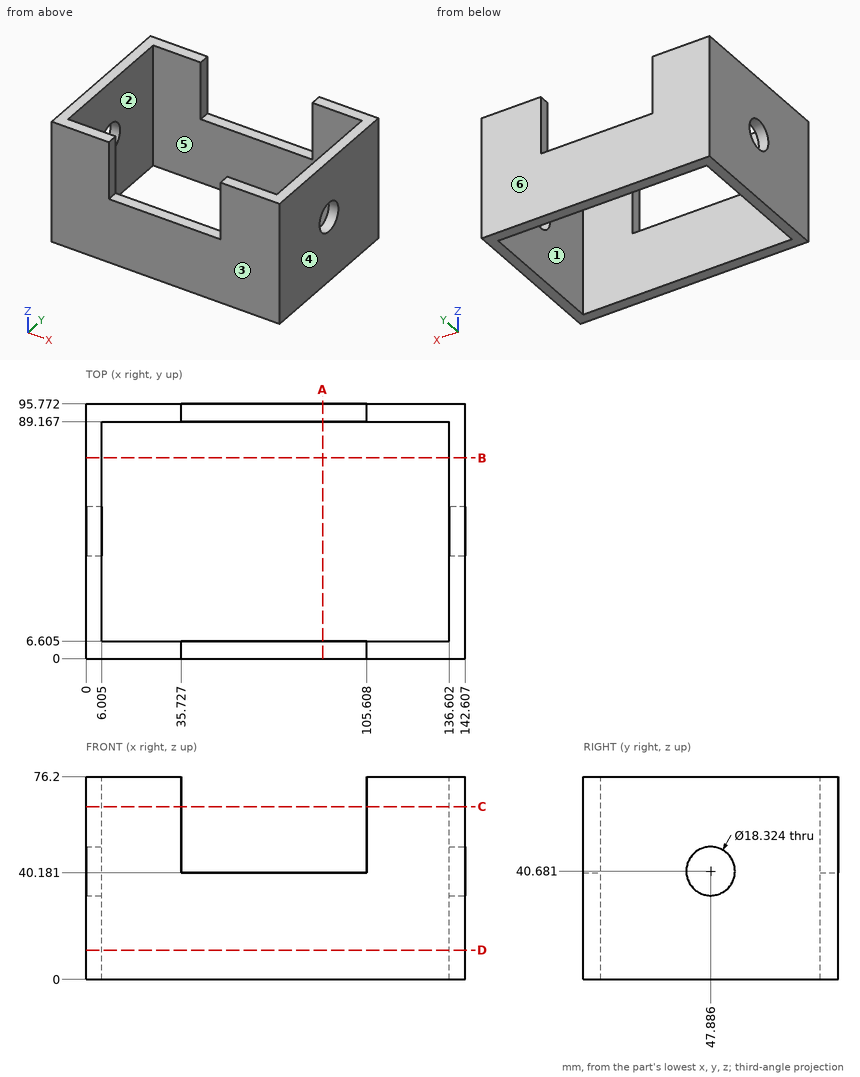
Source: three-view drawing plus pictorial views. Frame: mm from the lowest corner of the part. A direction names the side the tool comes from. Coordinates: 2 decimals unless noted, no trailing zeros. Loops run counter-clockwise (first coordinate to the right, second up) from the corner with the lowest first, then second, coordinate; pieces in that order, holes last. Notation, with made-up numbers: (-0.5, -30.5) - (33.5, -30.5) arc R20 cw to (33.5, 8.5) - close; hole circle Ø7 at (-8.75, 77.25). An arc over 180 degrees is marked (long way). One line per item, written item: value. Start each with the question number.
1. Ray query, L1, parallel to Y at x = 65, z = 22 (1 decimal); L2, parallel to X at y = 73, z = 64 (1 decimal); L3, parallel to Z at x = 47.5, y = 5. Return the intervals inside material, ascending.
2. Section C-C (z = 65). Return the cut outline in (x, y) (1 decimal).
3. Contact query for flat-ended pins moving along their axis: P1, Ø7.5, axis at x = 82, y = 2.5, coming from the +Z side; P2, Ø14.5, axis at y = 47.89, z = 40.68, coming from the +X side. Output: stop coordinate, or through.
4. Mould query, pull axis Y, two halves, no side actions, for the marked faces 1, 2, 3 and 4. Classes: pulls with the +Y half, pulls with the -Y half, needs draft (parallel to the pull), parting line crosses it, or undercut.
5. Section B-B (y = 75.5). Return the cut outline in (x, z) (1 decimal).
6. Section A-A (x = 89). Return the cut outline in (y, z) (1 decimal), and give its area (3 significant figures).
7. Section D-D (z = 11). Return the cut outline in (x, y) (1 decimal).
8. Set-up query: the marked faces 5 and 6. Return all of +Z, -Z, +X, -X, +Y, -Y with unobstructed straight access to the full face (end or side cutting, diameter ignored); none if empty.
Verdict:
1. L1: y = 0 to 6.6, 89.2 to 95.8
1. L2: x = 0 to 6, 136.6 to 142.6
1. L3: z = 0 to 40.18
2. outline: (0, 0) - (35.7, 0) - (35.7, 6.6) - (6, 6.6) - (6, 89.2) - (35.7, 89.2) - (35.7, 95.8) - (0, 95.8) - close; (105.6, 0) - (142.6, 0) - (142.6, 95.8) - (105.6, 95.8) - (105.6, 89.2) - (136.6, 89.2) - (136.6, 6.6) - (105.6, 6.6) - close
3. P1: stops at z = 40.18
3. P2: passes through
4. face 1: undercut
4. face 2: undercut
4. face 3: pulls with the -Y half
4. face 4: needs draft
5. outline: (0, 0) - (6, 0) - (6, 76.2) - (0, 76.2) - close; (136.6, 0) - (142.6, 0) - (142.6, 76.2) - (136.6, 76.2) - close
6. outline: (0, 0) - (6.6, 0) - (6.6, 40.2) - (0, 40.2) - close; (89.2, 0) - (95.8, 0) - (95.8, 40.2) - (89.2, 40.2) - close
6. area: 531 mm2
7. outline: (0, 0) - (142.6, 0) - (142.6, 95.8) - (0, 95.8) - close; hole (6, 6.6) - (136.6, 6.6) - (136.6, 89.2) - (6, 89.2) - close
8. face 5: +Z, -Z
8. face 6: +Z, -Z, +X, -X, +Y
